The drawing under review shows one solid part. Ordinate dimensions are in mm from its lowest x, y, z. A direction names the side the tool comes from. Coordinates: 2 decimals unless noted, no trailing zeros. Write each loop counter-clockwise with the first axis right and the second up, starting at its lowest first coordinate (ties: lowest second). Pieces come first, ordered by that corner, then holes.
1) For the marked faces 4 and 5, list the 3-axis set-ups (+Z, -Z, +X, -X, +Y, -Y) from which the entire face can be reached by the end or side of a thin tool; tool diameter is ignored.
2) We need section C-C on y = 6.5. Write out the cut boundary in (x, z), then the cut area to 3 significant figures.
3) Mouldability with a two-part tool opening along X and no side actions: class the marked faces 1, 2 and 3 as pulls with the +X half, pulls with the -X half, needs draft (parallel to the pull), parting line crosses it, or undercut.
4) We need section D-D on x = 16.5. Write out the cut boundary in (y, z).
5) We need section B-B on z = 40.5. Write out the cut boundary in (x, y), then the cut area to 3 significant figures.
6) To check wall thickness, follow line 1 along Z through (x, y) = (37, 6.25); line 2 along Z through (x, y) = (43, 9.25) (1 decimal); line 3 along X through (y, z) = (9.5, 110.5) (1 decimal). State the ranges of each line that lie inside material, in increasing order.
7) We need section A-A on x = 37. Write out the cut boundary in (y, z).
8) Insertion check: P1, Ø6, axis at y = 9, z = 14.5, coming from the +X side; P2, Ø1.5, axis at y = 3.5, z = 31.5, coming from the -X side; P3, Ø0.9, axis at y = 6.5, z = 32.5, coming from the +X side. Each pin has a flat end and moves straight along its axis. Give the tip position at first contact, or say it passes through.
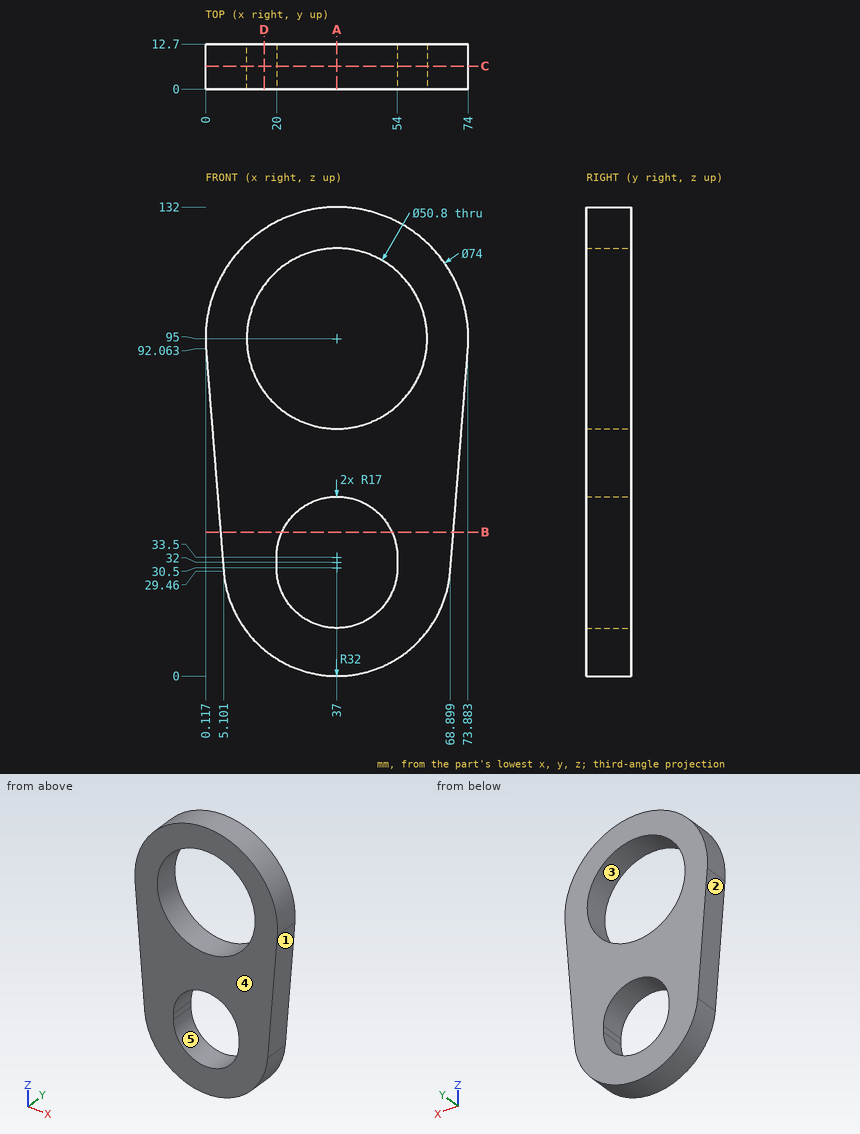
Result:
1. face 4: +Z, -Z, +X, -X, -Y
1. face 5: +Y, -Y
2. outline: (0.12, 92.06) - (5.1, 29.46) arc R32 ccw to (68.9, 29.46) - (73.88, 92.06) arc R37 ccw (long way) to start; hole circle Ø50.8 at (37, 95); hole (20, 30.5) arc R17 ccw to (54, 30.5) - (54, 33.5) arc R17 ccw to (20, 33.5) - close
2. area: 5,080 mm2
3. face 1: pulls with the +X half
3. face 2: pulls with the -X half
3. face 3: undercut
4. outline: (0, 7.43) - (12.7, 7.43) - (12.7, 80) - (0, 80) - close; (0, 110) - (12.7, 110) - (12.7, 125.8) - (0, 125.8) - close
5. outline: (4.22, 0) - (21.51, 0) - (21.51, 12.7) - (4.22, 12.7) - close; (52.49, 0) - (69.78, 0) - (69.78, 12.7) - (52.49, 12.7) - close
5. area: 439 mm2
6. line 1: z = 0 to 13.5, 50.5 to 69.6, 120.4 to 132
6. line 2: z = 0.6 to 14.6, 49.4 to 70.3, 119.7 to 131.5
6. line 3: x = 3.4 to 16.9, 57.1 to 70.6
7. outline: (0, 0) - (12.7, 0) - (12.7, 13.5) - (0, 13.5) - close; (0, 50.5) - (12.7, 50.5) - (12.7, 69.6) - (0, 69.6) - close; (0, 120.4) - (12.7, 120.4) - (12.7, 132) - (0, 132) - close
8. P1: stops at x = 65.53
8. P2: stops at x = 4.88
8. P3: stops at x = 69.18
